The model under review builds one solid part; all positions refer to its coordinate system, in mm. Face numbers are marked on the shaded views. Coordinates: 2 decimals unless noted, no trailing zeros. Order: outer loops, then holes, each group sorted by start corner. A loop starts at its lowest first (then second) coordinate and runs counter-clockwise, first axis right, second up. Notation, with made-up numbers: M 39,59 L 73,59 A36 cw 73,96 Z; hole C 13,64 d7. An arc over 180 degrees is marked long. Write each question's results on one line, items separated by ' | '.
from build123d import *

# Parameters (mm, degrees)
BOSS_EXTRUDE1_DEPTH = 10
CUT_EXTRUDE1_DEPTH  = 1
SKETCH7_R           = 2
SKETCH7_R_2         = 1.5
CUT_EXTRUDE2_DEPTH  = 1


with BuildPart() as part:
    # Sketch1 → Loft1 section 0
    with BuildSketch(Plane(origin=(0, 0, 0), x_dir=(1, 0, 0), z_dir=(0, 1, 0))):
        with BuildLine():
            Line((-20, 0), (0, 7.5))
            Line((0, 7.5), (20, 0))
            Line((20, 0), (0, -7.5))
            Line((0, -7.5), (-20, 0))
        make_face()
    # Sketch3 → Loft1 section 1
    with BuildSketch(Plane(origin=(0, 5, 0), x_dir=(-1, 0, 0), z_dir=(0, -1, 0))):
        with BuildLine():
            Line((0, 3.75), (-10, 0))
            Line((-10, 0), (0, -3.75))
            Line((0, -3.75), (10, 0))
            Line((10, 0), (0, 3.75))
        make_face()
    loft()

    # Sketch5 → Boss-Extrude1 (add)
    with BuildSketch(Plane(origin=(0, 0, 0), x_dir=(1, 0, 0), z_dir=(0, 1, 0))):
        with BuildLine():
            Line((-2, -2.236067977), (-2, 2.236067977))
            ThreePointArc((-2, 2.236067977), (3, 0), (-2, -2.236067977))
        make_face()
    extrude(amount=-BOSS_EXTRUDE1_DEPTH)

    # Sketch6 → Cut-Extrude1 (cut)
    with BuildSketch(Plane(origin=(0, 5, 0), x_dir=(-1, 0, 0), z_dir=(0, -1, 0))):
        with BuildLine():
            Line((-1.738096676, 2.445203457), (-1.378497417, 2.085604198))
            ThreePointArc((-1.378497417, 2.085604198), (1.767766953, 1.767766953), (2.085604198, -1.378497417))
            Line((2.085604198, -1.378497417), (2.445203457, -1.738096676))
            ThreePointArc((2.445203457, -1.738096676), (2.121320344, 2.121320344), (-1.738096676, 2.445203457))
        make_face()
        with BuildLine():
            Line((-2.445203457, 1.738096676), (-2.085604198, 1.378497417))
            ThreePointArc((-2.085604198, 1.378497417), (-1.767766953, -1.767766953), (1.378497417, -2.085604198))
            Line((1.378497417, -2.085604198), (1.738096676, -2.445203457))
            ThreePointArc((1.738096676, -2.445203457), (-2.121320344, -2.121320344), (-2.445203457, 1.738096676))
        make_face()
    extrude(amount=CUT_EXTRUDE1_DEPTH, mode=Mode.SUBTRACT)

    # Sketch7 → Cut-Extrude2 (cut)
    with BuildSketch(Plane(origin=(0, 5, 0), x_dir=(-1, 0, 0), z_dir=(0, -1, 0))):
        with Locations(Location((0, 0, 0), (0, 0, 180))):
            Circle(SKETCH7_R)
        with Locations(Location((0, 0, 0), (0, 0, 180))):
            Circle(SKETCH7_R_2, mode=Mode.SUBTRACT)
    extrude(amount=CUT_EXTRUDE2_DEPTH, mode=Mode.SUBTRACT)


solid = part.part
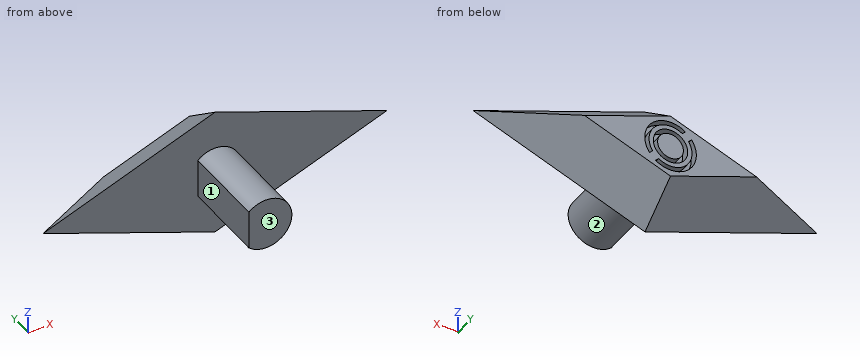
1) To check wall thickness, follow line 1 along Z through (x, y) = (0, 4.2); line 2 along Z through (x, y) = (0, 4.5) (3 decimals); line 3 along Y through (x, z) = (1, 6). State the ranges of each line that lie inside material, in increasing order.
Solutions:
line 1: -4.35 to -3, -2.5 to -2, -1.5 to 1.5, 2 to 2.5, 3 to 4.35 | line 2: -4.125 to -3, -2.5 to -2, -1.5 to 1.5, 2 to 2.5, 3 to 4.125 | line 3: 0 to 1.5
2) Take a section at A-A on y = -5.75. State the section outline as (x, z) points.
Solutions:
outline: M -2,-2.24 A3 ccw long -2,2.24 Z
3) For pin 1 (4 mm diameter, centred on x = -10, y = 1.5, fed in from +Z); pin 2 (4 mm diameter, centred on x = 5, z = 5.5, fed in from -Y); pin 3 (1.5 mm diameter, centred on x = -5.5, y = 2, fed in from +Z); pin 4 (2 mm diameter, centred on x = -14, z = 3.5, fed in from -Y), all flat-tipped, find the tip position at first contact; note any pin that passes through.
Solutions:
pin 1: z = 4.25 | pin 2: y = 0 | pin 3: z = 4.57 | pin 4: through
4) The part is to be moulded in two halves that separate along X. For the marked faces 1, 2 and 3, say which applies: pulls with the +X half, pulls with the -X half, needs draft (parallel to the pull), parting line crosses it, or undercut.
Solutions:
face 1: pulls with the -X half | face 2: parting line crosses it | face 3: needs draft
